Part model, mm, in its own coordinate system. Face numbers are marked on the shaded views. A direction names the side the tool comes from. Give positions to 0.01 mm unless a question says otherwise; leave off trailing zeros. Order: outer loops, then holes, each group sorted by start corner. A loop starts at its lowest first (then second) coordinate and runs counter-clockwise, first axis right, second up. Notation, with made-up numbers: M 3.5,65.25 L 34.5,65.25 A30 ccw 34.5,88.25 Z; hole C -18.5,55 d4. An arc over 180 degrees is marked long. Answer as a JSON object with one key per item and string values.
from build123d import *

# Parameters (mm, degrees)
SKETCH1_W           = 40
SKETCH1_H           = 80
SKETCH1_R           = 2
BOSS_EXTRUDE1_DEPTH = 21.25
SKETCH4_W           = 14.67
SKETCH4_H           = 80
BOSS_EXTRUDE3_DEPTH = 1
FILLET1_R           = 0.25
FILLET2_R           = 0.25
SKETCH2_W           = 10
SKETCH2_H           = 6
BOSS_EXTRUDE4_DEPTH = 6
SKETCH5_R           = 2.5
CUT_EXTRUDE1_DEPTH  = 53.896715399
SKETCH6_R           = 3
CUT_EXTRUDE2_DEPTH  = 6
FILLET3_R           = 1


with BuildPart() as part:
    # Sketch1 → Boss-Extrude1 (new body)
    with BuildSketch(Plane.XY):
        Rectangle(SKETCH1_W, SKETCH1_H)
        with Locations((12.3, 9.05)):
            Circle(SKETCH1_R, mode=Mode.SUBTRACT)
        with Locations((12.3, -9.05)):
            Circle(SKETCH1_R, mode=Mode.SUBTRACT)
        with Locations((-12.3, 9.05)):
            Circle(SKETCH1_R, mode=Mode.SUBTRACT)
        with Locations((-12.3, -9.05)):
            Circle(SKETCH1_R, mode=Mode.SUBTRACT)
    extrude(amount=BOSS_EXTRUDE1_DEPTH)

    # Sketch4 → Boss-Extrude3 (add)
    with BuildSketch(Plane(origin=(0, 0, 0), x_dir=(-1, 0, 0), z_dir=(0, 0, -1))):
        Rectangle(SKETCH4_W, SKETCH4_H)
    extrude(amount=BOSS_EXTRUDE3_DEPTH)

    # Fillet1
    fillet1_edges = [part.edges().sort_by_distance(p)[0] for p in [
        (7.335, 0, -1),
    ]]
    fillet(fillet1_edges, radius=FILLET1_R)

    # Fillet2
    fillet2_edges = [part.edges().sort_by_distance(p)[0] for p in [
        (-7.335, 0, -1),
    ]]
    fillet(fillet2_edges, radius=FILLET2_R)

    # Sketch2 → Boss-Extrude4 (add)
    with BuildSketch(Plane.XY.offset(21.25)):
        Polygon((-5, -13.05), (0, -13.05), (5, -13.05), (5, -7.05), (-5, -7.05), align=None)
        with Locations((0, 10.05)):
            Rectangle(SKETCH2_W, SKETCH2_H)
    extrude(amount=BOSS_EXTRUDE4_DEPTH)

    # Sketch5 → Cut-Extrude1 (cut, through all)
    with BuildSketch(Plane(origin=(0, 0, -1), x_dir=(-1, 0, 0), z_dir=(0, 0, -1))):
        with Locations((0, 29.5)):
            Circle(SKETCH5_R)
        with Locations(Location((0, -29.5, 0), (0, 0, 180))):
            Circle(SKETCH5_R)
    extrude(amount=-CUT_EXTRUDE1_DEPTH, mode=Mode.SUBTRACT)

    # Sketch6 → Cut-Extrude2 (cut)
    with BuildSketch(Plane.XY.offset(21.25)):
        with Locations((-12.3, 9.05)):
            Circle(SKETCH6_R)
        with Locations((12.3, 9.05)):
            Circle(SKETCH6_R)
        with Locations((12.3, -9.05)):
            Circle(SKETCH6_R)
        with Locations((-12.3, -9.05)):
            Circle(SKETCH6_R)
    extrude(amount=-CUT_EXTRUDE2_DEPTH, mode=Mode.SUBTRACT)

    # Fillet3
    fillet3_edges = [part.edges().sort_by_distance(p)[0] for p in [
        (5, -10.05, 27.25),
        (0, -7.05, 27.25),
        (-5, -10.05, 27.25),
        (0, -13.05, 27.25),
        (0, 13.05, 27.25),
        (-5, 10.05, 27.25),
        (0, 7.05, 27.25),
        (5, 10.05, 27.25),
    ]]
    fillet(fillet3_edges, radius=FILLET3_R)


solid = part.part
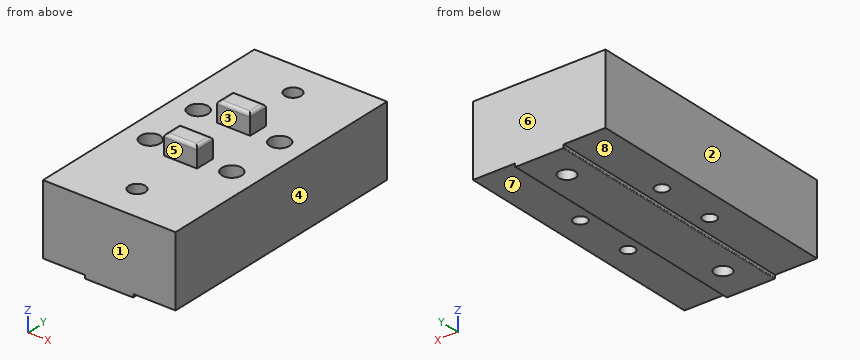
1. Two-plate mould, pull along Y, no slides. Class the marked faces 1, 2 and 3: +Y half, -Y half, draft (parallel to the pull), parting line (faces both ways), or undercut.
Worked answers:
{"face 1": "-Y half", "face 2": "draft", "face 3": "undercut"}
2. Cut at D-D on y = -9.05. State how many separate pieces and enclosed holes the cut face has, plus the area to 3 significant figures.
Worked answers:
{"separate pieces": "3", "enclosed holes": "0", "area": "730 mm^2"}
3. Cut at A-A on y = 29.5. Give the cut face in (x, z) (3 decimals).
Worked answers:
{"outline": "M -20,0 L -7.335,0 L -7.335,-0.75 A0.25 ccw -7.085,-1 L -2.5,-1 L -2.5,21.25 L -20,21.25 Z; M 2.5,-1 L 7.085,-1 A0.25 ccw 7.335,-0.75 L 7.335,0 L 20,0 L 20,21.25 L 2.5,21.25 Z"}
4. Pin check, flat tips, straight feed: P1, Ø6.5, axis at x = -12.5, y = -9, coming from the +Z side; P2, Ø6.5, axis at x = 0, y = -29.5, coming from the -Z side; P3, Ø3, axis at x = 12.3, y = 9.05, coming from the +Z side; P4, Ø5.5, axis at x = -12.3, y = 9.05, coming from the +Z side. Stop position of each tip, or through.
Worked answers:
{"P1": "stops at z = 21.25", "P2": "stops at z = -1", "P3": "passes through", "P4": "stops at z = 15.25"}
5. Probe line 1 along X through (y, z) = (-9.05, 4.5); line 2 along Y through (x, z) = (-12.3, 5.25); line 3 along Y through (x, z) = (12.3, 17.55). List the from-to ranges inside material, lowest first.
Worked answers:
{"line 1": "x = -20 to -14.3, -10.3 to 10.3, 14.3 to 20", "line 2": "y = -40 to -11.05, -7.05 to 7.05, 11.05 to 40", "line 3": "y = -40 to -12.05, -6.05 to 6.05, 12.05 to 40"}
6. Cut at B-B on x = -12.3. Give the cut face in (y, z).
Worked answers:
{"outline": "M -40,0 L -11.05,0 L -11.05,15.25 L -12.05,15.25 L -12.05,21.25 L -40,21.25 Z; M -7.05,0 L 7.05,0 L 7.05,15.25 L 6.05,15.25 L 6.05,21.25 L -6.05,21.25 L -6.05,15.25 L -7.05,15.25 Z; M 11.05,0 L 40,0 L 40,21.25 L 12.05,21.25 L 12.05,15.25 L 11.05,15.25 Z"}
7. Cut at C-C on z = 13.5. Give the cut face in (x, y).
Worked answers:
{"outline": "M -20,-40 L 20,-40 L 20,40 L -20,40 Z; hole C -12.3,-9.05 d4; hole C -12.3,9.05 d4; hole C 0,-29.5 d5; hole C 0,29.5 d5; hole C 12.3,-9.05 d4; hole C 12.3,9.05 d4"}
8. Which spindle directions (+Z, -Z, +X, -X, +Y, -Y) get a long thin tool onto all of the face, cutting with end or side? Do the marked faces 4, 5, 6, 7 and 8. Say none if no direction does.
Worked answers:
{"face 4": "+Z, -Z, +X, +Y, -Y", "face 5": "+Z, +X, -X, -Y", "face 6": "+Z, -Z, +X, -X, +Y", "face 7": "-Z, +X, +Y, -Y", "face 8": "-Z, -X, +Y, -Y"}
